Build history of the part. All positions in model axes, mm. Give positions to 0.01 mm unless a question says otherwise; leave off trailing zeros. Put each result on its own line as item: value. Start each with the question number.
Item 1: Flat gauge pins, fed straight in: pin 1 Ø1 at (y, z) = (-1, -2.5) entering from -X; pin 2 Ø0.6 at (y, z) = (-1, -4) entering from -X; pin 3 Ø1.5 at (x, z) = (15, -2) entering from +Y; pin 4 Ø0.8 at (x, y) = (55, -0.5) entering from -Z. Where does each tip first touch, or does it go through?
Item 2: Drill centre lines: line 1 along Z through (x, y) = (-52, -1.4); line 2 along Z through (x, y) = (-55.5, -0.95); line 3 along X through (y, z) = (-0.1, 4.75). Where is each one in solid material? Low to high.
Item 3: Slice it at A-A, the plane y = -1.2. Give the number of separate pieces and of enclosed holes in the cut face, plus the area to 3 significant figures.
```python
from build123d import *

# Parameters (mm, degrees)
F0_W     = 2.5
F0_H     = 4
F1_DEPTH = 2


# Not quite as in the source:
# - a feature names something its author has since deleted; it is built from what else it names


with BuildPart() as f1:
    # F0 (on Front) → F1 (new body)
    with BuildSketch(Plane.XZ):
        Polygon((56, -7.5), (85, -7.5), (85, 7.5), (-85, 7.5), (-85, -7.5), (-56, -7.5), (-56, 4.5), (-54.5, 4.5), (-54.5, -7.5), (-49.5, -7.5), (-49.5, 4.5), (-48, 4.5), (-48, -7.5), (-4, -7.5), (-4, 4.5), (-2.5, 4.5), (-2.5, -7.5), (2.5, -7.5), (2.5, 4.5), (4, 4.5), (4, -7.5), (48, -7.5), (48, 4.5), (49.5, 4.5), (49.5, -7.5), (54.5, -7.5), (54.5, 4.5), (56, 4.5), align=None)
        with Locations((-52, -3)):
            Rectangle(F0_W, F0_H, mode=Mode.SUBTRACT)
        with Locations((0, -3)):
            Rectangle(F0_W, F0_H, mode=Mode.SUBTRACT)
        with Locations((52, -3)):
            Rectangle(F0_W, F0_H, mode=Mode.SUBTRACT)
        Polygon((-85, -7.5), (-85, 7.5), (-100, 7.5), align=None)
        Polygon((85, 7.5), (85, -7.5), (100, 7.5), align=None)
        Polygon((-85, 7.5), (85, 7.5), (100, 7.5), (100, 16.5), (-100, 16.5), (-100, 7.5), align=None)
    extrude(amount=F1_DEPTH)


solid = f1.part
```
Values follow:
1. pin 1: x = -90.5
1. pin 2: x = -88.8
1. pin 3: y = 0
1. pin 4: z = 4.5
2. line 1: -7.5 to -5, -1 to 16.5
2. line 2: 4.5 to 16.5
2. line 3: -97.25 to 97.25
3. separate pieces: 1
3. enclosed holes: 3
3. area: 4,440 mm2
